Build history of the part. All positions in model axes, mm. Give positions to 0.01 mm unless a question says otherwise; leave off trailing zeros. Loops run counter-clockwise (first coordinate to the right, second up) from the corner with the lowest first, then second, coordinate; pieces in that order, holes last. Notation, with made-up numbers: M 0,67 L 26,67 A13 cw 26,82 Z; hole C -1,27 d4. An arc over 180 degrees is marked long. Answer as a JSON object with one key per item and string values. Group by question number.
1. Slice it at A-A (z = 0). List the corners of the cut face in (x, y), then the cut area to 3 significant figures.
2. Mould opens along X. For faces 1 (the face through (-219.693, 1.521, -4.506)), 2 (the face through (5, 3, -3)) say: released by +X, released by -X, zero draft, split by the parting line, or undercut.
3. Drop flat-ended pins along their axis: pin 1 Ø1.5 at (x, y) = (-378, 1.5) entering from -Z; pin 2 Ø0.9 at (y, z) = (1, 181) entering from -X; pin 3 Ø6.5 at (x, z) = (-331.06, 160) entering from -Y; pin 4 Ø10 at (x, z) = (223, 134) entering from -Y. Give the stop position or say it passes through.
4. Drill centre lines: line 1 along X through (y, z) = (0.9, -160); line 2 along Z through (x, y) = (331.06, 1.55); line 3 along Z through (x, y) = (-234, 1.9). Where is each one in solid material? Low to high. Write a range as [from, to].
from build123d import *

# Parameters (mm, degrees)
SKETCH2_R           = 3.5
BOSS_EXTRUDE1_DEPTH = 3
SKETCH3_R           = 15
CUT_EXTRUDE1_DEPTH  = 4
SKETCH4_R           = 5
CUT_EXTRUDE2_DEPTH  = 4


with BuildPart() as part:
    # Sketch2 → Boss-Extrude1 (new body)
    with BuildSketch(Plane(origin=(0, 0, 0), x_dir=(1, 0, 0), z_dir=(0, 1, 0))):
        Polygon((-375, 184), (375, 184), (375, 175), (384, 175), (384, -175), (375, -175), (375, -184), (-375, -184), (-375, -175), (-384, -175), (-384, 175), (-375, 175), align=None)
        with Locations((-331.06, 160)):
            Circle(SKETCH2_R, mode=Mode.SUBTRACT)
        with Locations((-331.06, -160)):
            Circle(SKETCH2_R, mode=Mode.SUBTRACT)
        with Locations((331.06, 160)):
            Circle(SKETCH2_R, mode=Mode.SUBTRACT)
        with Locations((331.06, -160)):
            Circle(SKETCH2_R, mode=Mode.SUBTRACT)
    extrude(amount=BOSS_EXTRUDE1_DEPTH)

    # Sketch3 → Cut-Extrude1 (cut, through all)
    with BuildSketch(Plane(origin=(0, 3, 0), x_dir=(1, 0, 0), z_dir=(0, 1, 0))):
        with Locations((-234, 0)):
            Circle(SKETCH3_R)
    extrude(amount=-CUT_EXTRUDE1_DEPTH, mode=Mode.SUBTRACT)

    # Sketch4 → Cut-Extrude2 (cut, through all)
    with BuildSketch(Plane(origin=(0, 3, 0), x_dir=(1, 0, 0), z_dir=(0, 1, 0))):
        with Locations((-234, 110)):
            Circle(SKETCH4_R)
    extrude(amount=-CUT_EXTRUDE2_DEPTH, mode=Mode.SUBTRACT)


solid = part.part
Established:
{
 "1": {"outline": "M -384,0 L -249,0 L -249,3 L -384,3 Z; M -219,0 L 384,0 L 384,3 L -219,3 Z", "area": "2,210 mm^2"},
 "2": {"face 1": "undercut", "face 2": "zero draft"},
 "3": {"pin 1": "stops at z = -175", "pin 2": "stops at x = -375", "pin 3": "passes through", "pin 4": "stops at y = 0"},
 "4": {"line 1": "x = [-384, -334.56], [-327.56, 327.56], [334.56, 384]", "line 2": "z = [-184, -163.5], [-156.5, 156.5], [163.5, 184]", "line 3": "z = [-184, -115], [-105, -15], [15, 184]"}
}
